```python
from build123d import *

# Parameters (mm, degrees)
SKETCH1_W           = 5.288
SKETCH1_H           = 5.288
BOSS_EXTRUDE1_DEPTH = 7
FILLET1_R           = 1


with BuildPart() as part:
    # Sketch1 → Boss-Extrude1 (new body)
    with BuildSketch(Plane.XY):
        with BuildLine():
            Line((6, 0), (6, -10))
            ThreePointArc((6, -10), (0, -16), (-6, -10))
            Line((-6, -10), (-6, 0))
            ThreePointArc((-6, 0), (0, 6), (6, 0))
        make_face()
        with Locations((0, -2.1)):
            Rectangle(SKETCH1_W, SKETCH1_H, mode=Mode.SUBTRACT)
    extrude(amount=BOSS_EXTRUDE1_DEPTH)

    # Sketch4 → Revolve1 (revolve)
    with BuildSketch(Plane(origin=(0, 0, 0), x_dir=(0, 0, -1), z_dir=(1, 0, 0)), mode=Mode.PRIVATE) as revolve1_sk:
        Polygon((-7, -13.625), (-11, -13.625), (-11, -14.264510891), (-12, -14.264510891), (-12, -13.625), (-17.25, -13.625), (-17.25, -14.264510891), (-18.25, -14.264510891), (-18.25, -13.625), (-27, -13.625), (-27, -10), (-7, -10), align=None)
    revolve(revolve1_sk.sketch.rotate(Axis((0, -10, 7), (0, 0, 1)), 270), axis=Axis((0, -10, 7), (0, 0, 1)))

    # Fillet1
    fillet1_edges = [part.edges().sort_by_distance(p)[0] for p in [
        (2.644, -2.1, 0),
        (0, 0.544, 0),
        (-2.644, -2.1, 0),
        (0, -4.744, 0),
    ]]
    fillet(fillet1_edges, radius=FILLET1_R)


solid = part.part
```
Part model, mm, in its own coordinate system. A direction names the side the tool comes from. Round coordinates to 2 decimals unless told otherwise and drop trailing zeros. Write each loop counter-clockwise with the first axis right and the second up, starting at its lowest first coordinate (ties: lowest second). Pieces come first, ordered by that corner, then holes. Notation, with made-up numbers: (20, 7.5) -> (36, 7.5) arc R19 cw to (36, 16.5) -> close; hole circle Ø8 at (19, -2). An arc over 180 degrees is marked (long way). Return JSON: item names as keys, results as strings. Group by question number.
Q1. Pin check, flat tips, straight feed: pin 1 (6 mm diameter, centred on x = 0.5, z = 13, fed in from +Y); pin 2 (1.5 mm diameter, centred on x = -2, z = 21.5, fed in from +Y); pin 3 (3 mm diameter, centred on x = 4, z = 12.5, fed in from -Y). Stop position of each tip, or through.
Q2. Mould opens along Y. For faces 1 (the cylindrical face through (-2.94, -2.05, 0.29)), 2 (the cylindrical face through (0.472, -13.594, 9.028)), 3 (the flat face through (-2.644, -2, 4)), 4 (the flat face through (0, -7, 0)) say: pulls with the +Y half, pulls with the -Y half, needs draft (parallel to the pull), parting line crosses it, or undercut.
Q3. Saw through at C-C on z = 23.75. Write the cut outline in (x, y) (3 decimals), plus the area to 3 significant figures.
Q4. Which spindle directions (+Z, -Z, +X, -X, +Y, -Y) get a long thin tool onto all of the face, cutting with end or side? Do faces 5 (the cylindrical face through (0.05, -5.04, 0.29)), 6 (the flat face through (0, -4.744, 4)), 7 (the cylindrical face through (0, 6, 3)), 8 (the cylindrical face through (0.924, -5.837, 17.757)). Say none if no direction does.
Q5. Probe L1, parallel to Y at x = 0, z = 2.25; L2, parallel to X at y = -3.75, z = 5.5; L3, parallel to Z at x = -2.5, y = -7.25. List the from-to ranges inside material, lowest first. Write a range as [from, to].
Q6. Saw through at D-D on y = -12.5. Write the cut outline in (x, z) (3 decimals), plus the area to 3 significant figures.
Q7. Saw through at A-A on y = -1. Write the cut outline in (x, z).
Answer:
{
 "1": {"pin 1": "y = -5.74", "pin 2": "y = -6.6", "pin 3": "y = -13.39"},
 "2": {"face 1": "undercut", "face 2": "parting line crosses it", "face 3": "undercut", "face 4": "needs draft"},
 "3": {"outline": "circle Ø7.25 at (0, -10)", "area": "41.3 mm2"},
 "4": {"face 5": "-Z", "face 6": "+Z, -Z", "face 7": "+Z, -Z, +Y", "face 8": "+Z"},
 "5": {"L1": "[-16, -4.74], [0.54, 6]", "L2": "[-6, -2.64], [2.64, 6]", "L3": "[0, 7], [11, 12], [17.25, 18.25]"},
 "6": {"outline": "(-5.454, 0) -> (5.454, 0) -> (5.454, 7) -> (2.625, 7) -> (2.625, 11) -> (3.455, 11) -> (3.455, 12) -> (2.625, 12) -> (2.625, 17.25) -> (3.455, 17.25) -> (3.455, 18.25) -> (2.625, 18.25) -> (2.625, 27) -> (-2.625, 27) -> (-2.625, 18.25) -> (-3.455, 18.25) -> (-3.455, 17.25) -> (-2.625, 17.25) -> (-2.625, 12) -> (-3.455, 12) -> (-3.455, 11) -> (-2.625, 11) -> (-2.625, 7) -> (-5.454, 7) -> close", "area": "185 mm2"},
 "7": {"outline": "(-6, 0) -> (-3.64, 0) arc R1 ccw to (-2.64, 1) -> (-2.64, 7) -> (-6, 7) -> close; (2.64, 1) arc R1 ccw to (3.64, 0) -> (6, 0) -> (6, 7) -> (2.64, 7) -> close"}
}
